Can you work these out from the model? Positions are in its coordinate system, mm. Round coordinates to 2 decimals unless told otherwise and drop trailing zeros. Loops run counter-clockwise (first coordinate to the right, second up) from the corner with the lowest first, then second, coordinate; pieces in that order, holes last. Notation, with made-up numbers: (56, 56) -> (111, 56) arc R27 ccw to (111, 78) -> close; hole circle Ø8 at (39, -21.5). An arc over 180 degrees is marked (long way). Write each question's results on one line, items separated by ' | '.
from build123d import *

# Parameters (mm, degrees)
BOSS_EXTRUDE1_DEPTH = 2570
FILLET1_R           = 1


with BuildPart() as part:
    # Sketch1 → Boss-Extrude1 (new body)
    with BuildSketch(Plane.XY):
        with BuildLine():
            Line((2.54, 0), (35.56, 0))
            ThreePointArc((35.56, 0), (37.356051224, -0.743948776), (38.1, -2.54))
            Line((38.1, -2.54), (38.1, -35.56))
            ThreePointArc((38.1, -35.56), (37.356051224, -37.356051224), (35.56, -38.1))
            Line((35.56, -38.1), (2.54, -38.1))
            ThreePointArc((2.54, -38.1), (0.743948776, -37.356051224), (0, -35.56))
            Line((0, -35.56), (0, -2.54))
            ThreePointArc((0, -2.54), (0.743948776, -0.743948776), (2.54, 0))
        make_face()
        with BuildLine():
            Line((5.3086, -2.7686), (32.7914, -2.7686))
            ThreePointArc((32.7914, -2.7686), (34.587451224, -3.512548776), (35.3314, -5.3086))
            Line((35.3314, -5.3086), (35.3314, -32.7914))
            ThreePointArc((35.3314, -32.7914), (34.587451224, -34.587451224), (32.7914, -35.3314))
            Line((32.7914, -35.3314), (5.3086, -35.3314))
            ThreePointArc((5.3086, -35.3314), (3.512548776, -34.587451224), (2.7686, -32.7914))
            Line((2.7686, -32.7914), (2.7686, -5.3086))
            ThreePointArc((2.7686, -5.3086), (3.512548776, -3.512548776), (5.3086, -2.7686))
        make_face(mode=Mode.SUBTRACT)
    extrude(amount=BOSS_EXTRUDE1_DEPTH)

    # Fillet1
    fillet1_edges = [part.edges().sort_by_distance(p)[0] for p in [
        (37.356051224, -37.356051224, 2570),
        (19.05, -38.1, 0),
        (0.743948776, -37.356051224, 0),
        (38.1, -19.05, 2570),
        (37.356051224, -0.743948776, 2570),
        (19.05, 0, 2570),
        (0.743948776, -0.743948776, 2570),
        (0, -19.05, 2570),
        (3.512548776, -34.587451224, 0),
        (19.05, -35.3314, 0),
        (34.587451224, -34.587451224, 0),
        (35.3314, -19.05, 0),
        (34.587451224, -3.512548776, 0),
        (19.05, -2.7686, 0),
        (3.512548776, -3.512548776, 0),
        (2.7686, -19.05, 0),
        (3.512548776, -34.587451224, 2570),
        (19.05, -35.3314, 2570),
        (34.587451224, -34.587451224, 2570),
        (35.3314, -19.05, 2570),
        (34.587451224, -3.512548776, 2570),
        (19.05, -2.7686, 2570),
        (3.512548776, -3.512548776, 2570),
        (2.7686, -19.05, 2570),
        (0.743948776, -37.356051224, 2570),
        (19.05, -38.1, 2570),
        (0, -19.05, 0),
        (0.743948776, -0.743948776, 0),
        (19.05, 0, 0),
        (37.356051224, -0.743948776, 0),
        (38.1, -19.05, 0),
        (37.356051224, -37.356051224, 0),
    ]]
    fillet(fillet1_edges, radius=FILLET1_R)


solid = part.part
1. Will these pins go through, and if not, where does the flat tip stop? pin 1 (10 mm diameter, centred on x = 32, y = -30, fed in from +Z); pin 2 (4 mm diameter, centred on x = 5, y = -9.5, fed in from +Z).
Final values:
pin 1: z = 2570 | pin 2: through
2. Please list where these lines run through material, in increasing order: line 1 (Y direction, x = 5, z = 1831.5); line 2 (X direction, y = -13, z = 611); line 3 (X direction, y = -4, z = 1753.5). Write a range as from..to.
Final values:
line 1: -38.1..-35.31, -2.79..0 | line 2: 0..2.77, 35.33..38.1 | line 3: 0..3.13, 34.97..38.1
3. If we section it at B-B (y = -20.5): List the corners of the cut face in (x, z) for me, then the cut area to 3 significant figures.
Final values:
outline: (0, 1) arc R1 ccw to (1, 0) -> (1.77, 0) arc R1 ccw to (2.77, 1) -> (2.77, 2569) arc R1 ccw to (1.77, 2570) -> (1, 2570) arc R1 ccw to (0, 2569) -> close; (35.33, 1) arc R1 ccw to (36.33, 0) -> (37.1, 0) arc R1 ccw to (38.1, 1) -> (38.1, 2569) arc R1 ccw to (37.1, 2570) -> (36.33, 2570) arc R1 ccw to (35.33, 2569) -> close | area: 14,200 mm2
4. If we section it at A-A (x = 22): List the corners of the cut face in (y, z) for me, then the cut area to 3 significant figures.
Final values:
outline: (-38.1, 1) arc R1 ccw to (-37.1, 0) -> (-36.33, 0) arc R1 ccw to (-35.33, 1) -> (-35.33, 2569) arc R1 ccw to (-36.33, 2570) -> (-37.1, 2570) arc R1 ccw to (-38.1, 2569) -> close; (-2.77, 1) arc R1 ccw to (-1.77, 0) -> (-1, 0) arc R1 ccw to (0, 1) -> (0, 2569) arc R1 ccw to (-1, 2570) -> (-1.77, 2570) arc R1 ccw to (-2.77, 2569) -> close | area: 14,200 mm2
5. If we section it at C-C (z = 2036): List the corners of the cut face in (x, y) for me, then the cut area to 3 significant figures.
Final values:
outline: (0, -35.56) arc R2.54 ccw to (2.54, -38.1) -> (35.56, -38.1) arc R2.54 ccw to (38.1, -35.56) -> (38.1, -2.54) arc R2.54 ccw to (35.56, 0) -> (2.54, 0) arc R2.54 ccw to (0, -2.54) -> close; hole (2.77, -32.79) arc R2.54 ccw to (5.31, -35.33) -> (32.79, -35.33) arc R2.54 ccw to (35.33, -32.79) -> (35.33, -5.31) arc R2.54 ccw to (32.79, -2.77) -> (5.31, -2.77) arc R2.54 ccw to (2.77, -5.31) -> close | area: 391 mm2
